from build123d import *

# Parameters (mm, degrees)
F1_DEPTH = 11.5
F2_D     = 2.8
F3_R     = 2.99999


# Not quite as in the source:
# - a fillet or chamfer is up to 0.001 mm smaller than in the source, because OpenCascade refuses the exact size


with BuildPart() as f1:
    # F0 (on Top) → F1 (new body)
    with BuildSketch(Plane.XY):
        with BuildLine():
            Line((-61, -5.1), (24, -5.1))
            Line((24, -5.1), (24, -3.5))
            Line((24, -3.5), (3, -3.5))
            Line((3, -3.5), (3, 0))
            ThreePointArc((3, 0), (0, 3), (-3, 0))
            Line((-3, 0), (-3, -3.5))
            Line((-3, -3.5), (-55, -3.5))
            Line((-55, -3.5), (-55, 0))
            ThreePointArc((-55, 0), (-58, 3), (-61, 0))
            Line((-61, 0), (-61, -0.5))
            Line((-61, -0.5), (-71.5, -0.5))
            Line((-71.5, -0.5), (-71.5, 1.1))
            Line((-71.5, 1.1), (-76.5, -0.5))
            Line((-76.5, -0.5), (-76.5, -2.1))
            Line((-76.5, -2.1), (-61, -2.1))
            Line((-61, -2.1), (-61, -5.1))
        make_face()
    extrude(amount=F1_DEPTH)

    # F2 (through all)
    with Locations(Plane(origin=(0, 0, 0), x_dir=(1, 0, 0), z_dir=(0, 0, -1))):
        with Locations((-58, 0), (0, 0)):
            Hole(F2_D / 2)

    # F3 (radius 3 in the source; OpenCascade refuses exactly that, so slightly less here)
    f3_edges = [f1.edges().sort_by_distance(p)[0] for p in [
        (-61, -2.1, 5.75),
    ]]
    fillet(f3_edges, radius=F3_R)


solid = f1.part
Could you check a few things on this model? Use its own coordinates, in mm. A direction names the side the tool comes from. Give positions to 0.01 mm unless a question says otherwise; leave off trailing zeros. Order: outer loops, then holes, each group sorted by start corner. A loop starts at its lowest first (then second) coordinate and runs counter-clockwise, first axis right, second up.
1. Suppose I cut it at C-C (x = -39.5). List the corners of the cut face in (y, z) for me, plus the area to 3 significant figures.
2. For faces 1 (the flat face through (-29, -3.5, 6)), 2 (the flat face through (-70, -2.1, 6)), 3 (the flat face through (3, -2, 6)), which set-ups out of +Z, -Z, +X, -X, +Y, -Y let a thin tool reach every point of the face, with its end or its side?
3. I need wall thicknesses on L1, parallel to X at y = -1.5, z = 3; L2, parallel to Y at x = -58, z = 4.25; L3, parallel to Y at x = -38.5, z = 7.75. Which ranges of each line are inside material? Lowest first, please.
4. Will these pins go through, and if not, where does the flat tip stop? P1, Ø1.5, axis at x = -36, z = 4, coming from the +Y side; P2, Ø1.8, axis at y = -1.5, z = 7.5, coming from the +X side; P3, Ø5, axis at x = -66, z = 4.5, coming from the +Y side.
5. We'd pull the mould along Y, two halves only. Please class faces 4 (the flat face through (-55, -2, 6)), 5 (the cylindrical face through (0, 3, 6)), 6 (the cylindrical face through (-59.335, -0.421, 5.831)): pulls with the +Y half, pulls with the -Y half, needs draft (parallel to the pull), parting line crosses it, or undercut.
6. Suppose I cut it at A-A (x = -58). List the corners of the cut face in (y, z) for me.
7. Suppose I cut it at B-B (z = 6). Give the number of separate pieces and of enclosed holes in the cut face, plus the area to 3 significant figures.
Solved:
1. outline: (-5.1, 0) - (-3.5, 0) - (-3.5, 11.5) - (-5.1, 11.5) - close
1. area: 18.4 mm2
2. face 1: +Z, -Z, +Y
2. face 2: +Z, -Z, -X, -Y
2. face 3: +Z, -Z, +X, +Y
3. L1: x = -76.5 to -55, -3 to 3
3. L2: y = -5.1 to -1.4, 1.4 to 3
3. L3: y = -5.1 to -3.5
4. P1: stops at y = -3.5
4. P2: stops at x = 3
4. P3: stops at y = -0.5
5. face 4: needs draft
5. face 5: pulls with the +Y half
5. face 6: undercut
6. outline: (-5.1, 0) - (-1.4, 0) - (-1.4, 11.5) - (-5.1, 11.5) - close; (1.4, 0) - (3, 0) - (3, 11.5) - (1.4, 11.5) - close
7. separate pieces: 1
7. enclosed holes: 2
7. area: 225 mm2
